The listing builds one solid part. Answer for the finished solid, in the listing's coordinates (mm). A direction names the side the tool comes from. Give positions to 0.01 mm unless a question says otherwise; leave off trailing zeros. Write each loop counter-clockwise with the first axis right and the second up, starting at its lowest first coordinate (ties: lowest second). Pieces come first, ordered by that corner, then holes. Notation, with made-up numbers: (46.5, -28) -> (83.5, -28) arc R23 cw to (83.5, 1) -> close; hole circle Ø8 at (84, 24.25). An arc over 180 degrees is marked (long way). One line per question, with ' | ' between items.
from build123d import *

# Parameters (mm, degrees)
BOSS_EXTRU_1_DEPTH      = 4
BOSS_EXTRU_1_DEPTH_BACK = 4
ESQUISSE1_R             = 4
BOSS_EXTRU_2_DEPTH      = 10
BOSS_EXTRU_2_DEPTH_BACK = 10
ESQUISSE2_R             = 1


with BuildPart() as part:
    # Esquisse1 → Boss.-Extru.1 (new, two sides: drawn at the far end of the back side and taken through both)
    with BuildSketch(Plane.XY.offset(-BOSS_EXTRU_1_DEPTH_BACK)):
        Circle(ESQUISSE1_R)
    extrude(amount=BOSS_EXTRU_1_DEPTH + BOSS_EXTRU_1_DEPTH_BACK)

    # Esquisse2 → Boss.-Extru.2 (add, two sides: drawn at the far end of the back side and taken through both)
    with BuildSketch(Plane.XY.offset(-BOSS_EXTRU_2_DEPTH_BACK)):
        Circle(ESQUISSE2_R)
    extrude(amount=BOSS_EXTRU_2_DEPTH + BOSS_EXTRU_2_DEPTH_BACK)


solid = part.part
Item 1: Consider line 1 (Z direction, x = 3.75, y = 0.75); line 2 (Y direction, x = -2.5, z = 0); line 3 (Y direction, x = 0.75, z = 5.5). Determine where each line is inside the solid, lowest interval first. Write a range as [from, to].
Answers below:
line 1: [-4, 4] | line 2: [-3.12, 3.12] | line 3: [-0.66, 0.66]
Item 2: Find section C-C (z = -7.5). Write down the section's boundary in (x, y), then the cut area to 3 significant figures.
Answers below:
outline: circle Ø2 at (0, 0) | area: 3.14 mm²
Item 3: A flat-ended cylindrical pin translates along its axis: pin 1 (2 mm diameter, centred on y = -2.5, z = 3.5, fed in from +X). Find the tip coordinate at first contact, or state that the pin passes through.
Answers below:
pin 1: x = 3.71
Item 4: Find section A-A (y = 0). Write down the section's boundary in (x, z), then the cut area to 3 significant figures.
Answers below:
outline: (-4, -4) -> (-1, -4) -> (-1, -10) -> (1, -10) -> (1, -4) -> (4, -4) -> (4, 4) -> (1, 4) -> (1, 10) -> (-1, 10) -> (-1, 4) -> (-4, 4) -> close | area: 88.0 mm²
Item 5: Find section D-D (z = -1.75). Write down the section's boundary in (x, y).
Answers below:
outline: circle Ø8 at (0, 0)
Item 6: A tool of negligible diameter and unlimited length cuts with its end or side. For faces 1 (the face through (1, -1, 4)), 2 (the face through (1, -1, -4)), 3 (the face through (0, 0, -10)), from which of +Z, -Z, +X, -X, +Y, -Y can it reach the whole face along a straight path? Write none if from no direction.
Answers below:
face 1: +Z | face 2: -Z | face 3: -Z, +X, -X, +Y, -Y
